Design review of the part shown in the three views and the two pictorial views. Dimensions are in mm from the part's minimum x, y and z. A direction names the side the tool comes from. Coordinates: 2 decimals unless noted, no trailing zeros. Loops run counter-clockwise (first coordinate to the right, second up) from the corner with the lowest first, then second, coordinate; pieces in that order, holes last. Notation, with made-up numbers: M 5.25,-26 L 31.25,-26 A23 ccw 31.25,-5 Z; hole C 5.5,70 d4. An arc over 180 degrees is marked long. Use one line per item in the form item = value.
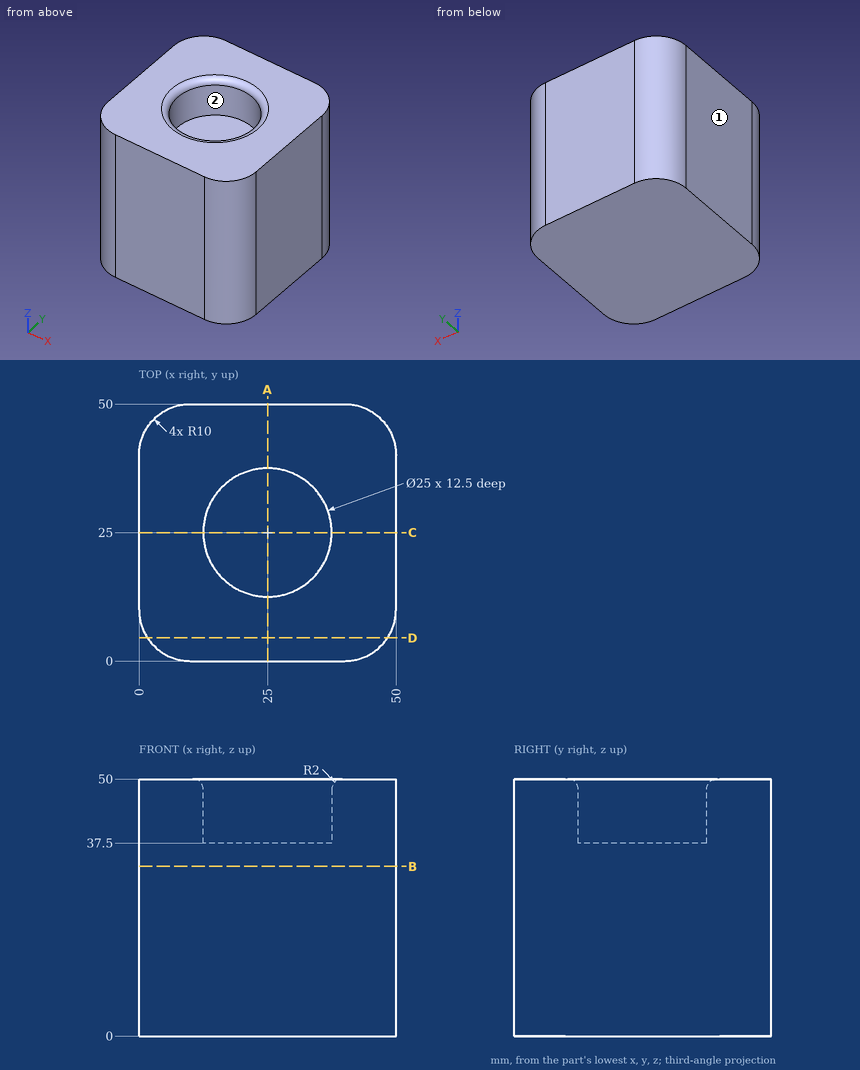
1. Wall thickness on line 1 along Y through (x, z) = (25, 40.5); line 2 along Y through (x, z) = (9.5, 35); line 3 along Z through (x, y) = (28, 22): over which ranges is each line inside the solid? List them lowest first. Write a range as from..to.
Response values:
line_1 = 0..12.5, 37.5..50
line_2 = 0.01..49.99
line_3 = 0..37.5
2. Add section D-D (y = 4.5). State the section outline as (x, z) points.
Response values:
outline = M 1.65,0 L 48.35,0 L 48.35,50 L 1.65,50 Z
3. Add section A-A (x = 25). State the section outline as (y, z) points, then the cut area to 3 significant figures.
Response values:
outline = M 0,0 L 50,0 L 50,50 L 39.5,50 A2 ccw 37.5,48 L 37.5,37.5 L 12.5,37.5 L 12.5,48 A2 ccw 10.5,50 L 0,50 Z
area = 2,190 mm^2
4. Machinability: for the marked faces 1 and 2, which of the approach directions +Z, -Z, +X, -X, +Y, -Y give a long, thin tool a straight path to every point of the face, cutting with its end or side? Answer none if there is none.
Response values:
face_1 = +Z, -Z, -X, +Y, -Y
face_2 = +Z
5. Add section B-B (z = 33). State the section outline as (x, y) points.
Response values:
outline = M 0,10 A10 ccw 10,0 L 40,0 A10 ccw 50,10 L 50,40 A10 ccw 40,50 L 10,50 A10 ccw 0,40 Z
